```python
from build123d import *

# Parameters (mm, degrees)
F1_W   = 1
F1_H   = 1
F1_H_2 = 3


with BuildPart() as f2:
    # F1 (on Top) → F2 (revolve)
    with BuildSketch(Plane.XY):
        with Locations((5.8, 19.201042)):
            Rectangle(F1_W, F1_H)
        Polygon((5.3, 18.701042), (5.3, -5.298958), (6.3, -5.298958), (6.3, 12.701042), (6.3, 15.701042), (6.3, 18.701042), align=None)
        Polygon((6.3, 19.701042), (6.3, 18.701042), (7, 18.701042), (17.1, 18.701042), (17.1, 19.701042), align=None)
        with BuildLine():
            Line((7, 18.701042), (6.3, 18.701042))
            Line((6.3, 18.701042), (6.3, 15.701042))
            Line((6.3, 15.701042), (7.3, 15.701042))
            ThreePointArc((7.3, 15.701042), (6.489082, 17.13495), (7, 18.701042))
        make_face()
        with Locations((6.8, 14.201042)):
            Rectangle(F1_W, F1_H_2)
    revolve(axis=Axis((0, 5.007949, 0), (0, 1, 0)))


solid = f2.part
```
For this review, take the finished solid that the model builds, in its own axes (mm). A direction names the side the tool comes from. Round coordinates to 2 decimals unless told otherwise and drop trailing zeros. Write each loop counter-clockwise with the first axis right and the second up, starting at its lowest first coordinate (ties: lowest second). Pieces come first, ordered by that corner, then holes.
1) For line 1 along Z through (x, y) = (0, 8.25); line 2 along X through (y, z) = (14.25, 0), list the stretches that pass through material, from the lowest coordinate up.
Answer below:
line 1: z = -6.3 to -5.3, 5.3 to 6.3
line 2: x = -7.3 to -5.3, 5.3 to 7.3
2) Take a section at D-D on z = 15.5. Give the boundary of the cut face in (x, y), then the cut area to 3 significant figures.
Answer below:
outline: (-7.22, 18.7) - (7.22, 18.7) - (7.22, 19.7) - (-7.22, 19.7) - close
area: 14.4 mm2
3) Take a section at C-C on y = 9.25. Give the boundary of the cut face in (x, z).
Answer below:
outline: circle Ø12.6 at (0, 0); hole circle Ø10.6 at (0, 0)
4) Take a section at A-A on x = 0. Give the boundary of the cut face in (y, z).
Answer below:
outline: (-5.3, -6.3) - (12.7, -6.3) - (12.7, -7.3) - (15.7, -7.3) arc R2.04 cw to (18.7, -7) - (18.7, -17.1) - (19.7, -17.1) - (19.7, -5.3) - (-5.3, -5.3) - close; (-5.3, 5.3) - (19.7, 5.3) - (19.7, 17.1) - (18.7, 17.1) - (18.7, 7) arc R2.04 cw to (15.7, 7.3) - (12.7, 7.3) - (12.7, 6.3) - (-5.3, 6.3) - close
5) Insertion check: pin 1 Ø8 at (x, y) = (7.5, 13.5) entering from +Z; pin 2 Ø9.5 at (x, z) = (0, 0) entering from +Y; pin 3 Ø8 at (x, y) = (0.5, 10.5) entering from -Z; pin 4 Ø12 at (x, y) = (-8, 9) entering from +Z. Each pin has a flat end and moves straight along its axis. Give the tip position at first contact, or say it passes through.
Answer below:
pin 1: stops at z = 6.41
pin 2: passes through
pin 3: stops at z = -7.3
pin 4: stops at z = 6.52
6) Mouldability with a two-part tool opening along Z and no side actions: class faces 3 (the face through (4, 19.701, -4)), 4 (the face through (-5, 3.83, 3.83)), 5 (the face through (4.896, 7.026, 2.03)) as +Z half, -Z half, draft (parallel to the pull), parting line (faces both ways), or undercut.
Answer below:
face 3: draft
face 4: parting line
face 5: undercut
7) Machinability: for faces 1 (the face through (6.963, 14.222, -2.193)), 2 (the face through (16.31, 19.21, -5.14)), which of the approach directions +Z, -Z, +X, -X, +Y, -Y give a long, thin tool a straight path to every point of the face, cutting with its end or side? Answer none if there is none.
Answer below:
face 1: -Y
face 2: +Y, -Y
8) Take a section at B-B on z = 0. Give the boundary of the cut face in (x, y).
Answer below:
outline: (-17.1, 18.7) - (-7, 18.7) arc R2.04 cw to (-7.3, 15.7) - (-7.3, 12.7) - (-6.3, 12.7) - (-6.3, -5.3) - (-5.3, -5.3) - (-5.3, 19.7) - (-17.1, 19.7) - close; (5.3, -5.3) - (6.3, -5.3) - (6.3, 12.7) - (7.3, 12.7) - (7.3, 15.7) arc R2.04 cw to (7, 18.7) - (17.1, 18.7) - (17.1, 19.7) - (5.3, 19.7) - close
